from build123d import *

# Parameters (mm, degrees)
F0_W     = 30
F0_H     = 50
F1_DEPTH = 2.5
F2_W     = 2.5
F2_H     = 50
F3_DEPTH = 10
F4_W     = 20
F4_H     = 50
F4_R     = 3
F5_DEPTH = 2.5
F6_W     = 4
F6_H     = 2.5
F7_DEPTH = 12.5
F8_W     = 10
F8_H     = 2.5
F9_DEPTH = 12.5


with BuildPart() as f1:
    # F0 (on Top) → F1 (new body)
    with BuildSketch(Plane.XY):
        with Locations((0, 0.874573)):
            Rectangle(F0_W, F0_H)
    extrude(amount=F1_DEPTH)

    # F2 (on Top) → F3 (join)
    with BuildSketch(Plane.XY):
        with Locations((16.25, 0.874573)):
            Rectangle(F2_W, F2_H)
        with Locations((-16.25, 0.874573)):
            Rectangle(F2_W, F2_H)
    extrude(amount=F3_DEPTH)

    # F4 (on face) → F5 (join)
    with BuildSketch(Plane.XY.offset(10)):
        with Locations((25, 0.874573)):
            Rectangle(F4_W, F4_H)
        with Locations((25, -11.125427)):
            Circle(F4_R, mode=Mode.SUBTRACT)
        with Locations((25, 12.874573)):
            Circle(F4_R, mode=Mode.SUBTRACT)
        with Locations((-25, 0.874573)):
            Rectangle(F4_W, F4_H)
        with Locations((-25, -11.125427)):
            Circle(F4_R, mode=Mode.SUBTRACT)
        with Locations((-25, 12.874573)):
            Circle(F4_R, mode=Mode.SUBTRACT)
    extrude(amount=F5_DEPTH)

    # F6 (on Top) → F7 (join, through all)
    with BuildSketch(Plane.XY):
        with Locations((-4, 27.124573)):
            Rectangle(F6_W, F6_H)
    extrude(amount=F7_DEPTH)

    # F8 (on Top) → F9 (join, through all)
    with BuildSketch(Plane.XY):
        with Locations((0, -25.375427)):
            Rectangle(F8_W, F8_H)
    extrude(amount=F9_DEPTH)


solid = f1.part
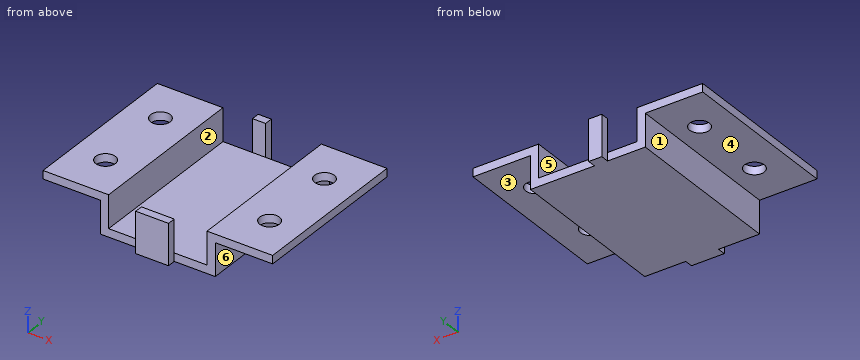
The listing builds one solid part. Answer for the finished solid, in the listing's coordinates (mm). Face numbers are marked on the shaded views. A direction names the side the tool comes from. Coordinates: 2 decimals unless noted, no trailing zeros. Write each loop counter-clockwise with the first axis right and the second up, starting at its lowest first coordinate (ties: lowest second). Pieces come first, ordered by that corner, then holes. Notation, with made-up numbers: (58, 0) -> (109, 0) arc R13 cw to (109, 21) -> close; hole circle Ø4 at (43.5, 78.5). An arc over 180 degrees is marked (long way). One line per question, with ' | ' between items.
1. Section D-D (z = 1.75) is taken. Determine the outline of the cut face in (x, y), and give its area (4 significant figures).
Verdict:
outline: (-17.5, -24.13) -> (-5, -24.13) -> (-5, -26.63) -> (5, -26.63) -> (5, -24.13) -> (17.5, -24.13) -> (17.5, 25.87) -> (-2, 25.87) -> (-2, 28.37) -> (-6, 28.37) -> (-6, 25.87) -> (-17.5, 25.87) -> close | area: 1,785 mm^2
2. Straight lines are drawn through the part: line 1 (Y direction, x = 25, z = 11.6); line 2 (X direction, y = 19, z = 9.5); line 3 (X direction, y = -13, z = 10.5). For each, find the intervals that lie inside material, in ascending order.
Verdict:
line 1: y = -24.13 to -14.13, -8.13 to 9.87, 15.87 to 25.87 | line 2: x = -17.5 to -15, 15 to 17.5 | line 3: x = -35 to -27.34, -22.66 to -15, 15 to 22.66, 27.34 to 35
3. Section A-A (z = 8) is taken. Determine the outline of the cut face in (x, y).
Verdict:
outline: (-17.5, -24.13) -> (-15, -24.13) -> (-15, 25.87) -> (-17.5, 25.87) -> close; (-6, 25.87) -> (-2, 25.87) -> (-2, 28.37) -> (-6, 28.37) -> close; (-5, -26.63) -> (5, -26.63) -> (5, -24.13) -> (-5, -24.13) -> close; (15, -24.13) -> (17.5, -24.13) -> (17.5, 25.87) -> (15, 25.87) -> close
4. Section B-B (x = -25) is taken. Determine the outline of the cut face in (y, z), and give its area (3 significant figures).
Verdict:
outline: (-24.13, 10) -> (-14.13, 10) -> (-14.13, 12.5) -> (-24.13, 12.5) -> close; (-8.13, 10) -> (9.87, 10) -> (9.87, 12.5) -> (-8.13, 12.5) -> close; (15.87, 10) -> (25.87, 10) -> (25.87, 12.5) -> (15.87, 12.5) -> close | area: 95.0 mm^2
5. Which of the six approach directions +Z, -Z, +X, -X, +Y, -Y give full straight-line access (tool end or side, diameter ignored) to the marked faces 4, 5 and 6?
Verdict:
face 4: -Z, -X, +Y, -Y | face 5: +Z, +Y, -Y | face 6: -Z, +X, +Y, -Y
6. For a pull along X with two mould halves and no side action, classify the marked faces 1, 2 and 3 as released by +X, released by -X, zero draft, split by the parting line, or undercut.
Verdict:
face 1: released by -X | face 2: undercut | face 3: zero draft
7. Given pin 1 Ø1.5 at (x, y) = (19.5, 12) entering from -Z; pin 2 Ø3 at (y, z) = (0.5, 5) entering from -X; pin 3 Ø9 at (x, y) = (-6.5, -3.5) entering from +Z, each flat-ended and moving along its own axis, determine where each tip first touches the part or whether it passes through.
Verdict:
pin 1: stops at z = 10 | pin 2: stops at x = -17.5 | pin 3: stops at z = 2.5
8. Section C-C (z = 11.5) is taken. Determine the outline of the cut face in (x, y), and give its area (3 significant figures).
Verdict:
outline: (-35, -24.13) -> (-15, -24.13) -> (-15, 25.87) -> (-35, 25.87) -> close; (-6, 25.87) -> (-2, 25.87) -> (-2, 28.37) -> (-6, 28.37) -> close; (-5, -26.63) -> (5, -26.63) -> (5, -24.13) -> (-5, -24.13) -> close; (15, -24.13) -> (35, -24.13) -> (35, 25.87) -> (15, 25.87) -> close; hole circle Ø6 at (-25, -11.13); hole circle Ø6 at (-25, 12.87); hole circle Ø6 at (25, -11.13); hole circle Ø6 at (25, 12.87) | area: 1,920 mm^2
